Read the model definition and answer for the solid it produces. Units are mm, in the model's axes. A direction names the side the tool comes from. Give positions to 0.01 mm unless a question says otherwise; leave off trailing zeros. Order: outer loops, then holes, each group sorted by start corner. A loop starts at its lowest first (then second) coordinate and runs counter-clockwise, first axis right, second up. Notation, with made-up numbers: (36.5, -14) - (87.5, -14) arc R25 cw to (87.5, 2) - close; hole circle Ø5 at (-13, -7.75). An arc over 180 degrees is marked (long way). Write each question's results on one line, items separated by ' | '.
from build123d import *

# Parameters (mm, degrees)
BOSS_EXTRUDE1_DEPTH      = 1.5
BOSS_EXTRUDE1_DEPTH_BACK = 1.5
SKETCH1_R                = 8.5
SKETCH1_R_2              = 2.3
SKETCH2_W                = 3
SKETCH2_H                = 2.6
SKETCH2_W_2              = 2.6
SKETCH2_H_2              = 3
CUT_EXTRUDE1_DEPTH       = 13.389511693


with BuildPart() as part:
    # Sketch1 → Boss-Extrude1 (new, two sides: drawn at the far end of the back side and taken through both)
    with BuildSketch(Plane(origin=(0, 0, 0), x_dir=(1, 0, 0), z_dir=(0, 1, 0)).offset(-BOSS_EXTRUDE1_DEPTH_BACK)):
        with Locations(Location((0, 0, 0), (0, 0, 270))):
            Circle(SKETCH1_R)
        with Locations(Location((0, 0, 0), (0, 0, 270))):
            Circle(SKETCH1_R_2, mode=Mode.SUBTRACT)
    extrude(amount=BOSS_EXTRUDE1_DEPTH + BOSS_EXTRUDE1_DEPTH_BACK)

    # Sketch2 → Cut-Extrude1 (cut, through all)
    with BuildSketch(Plane(origin=(0, 1.5, 0), x_dir=(1, 0, 0), z_dir=(0, 1, 0))):
        with Locations((-7, 0)):
            Rectangle(SKETCH2_W, SKETCH2_H)
        with Locations((0, -7)):
            Rectangle(SKETCH2_W_2, SKETCH2_H_2)
        with Locations((0, 7)):
            Rectangle(SKETCH2_W_2, SKETCH2_H_2)
        with Locations((7, 0)):
            Rectangle(SKETCH2_W, SKETCH2_H)
    extrude(amount=-CUT_EXTRUDE1_DEPTH, mode=Mode.SUBTRACT)


solid = part.part
(1) Each of these flat-tipped pins is pushed along its axis until it touches: pin 1 (1.5 mm diameter, centred on x = -6.5, y = -0.5, fed in from +Z); pin 2 (0.8 mm diameter, centred on x = 0, y = -0.5, fed in from +Z); pin 3 (1.5 mm diameter, centred on y = 0, z = -6.5, fed in from +X). Where does it stop, or does it pass through?
Conclusion:
pin 1: z = 6.26 | pin 2: z = 5.5 | pin 3: x = 6.26
(2) The mould has two halves that part along X. Classify faces 6 (the face through (5.96, -0.02, 6.06)), 7 (the face through (-7, 0, -1.3)), 8 (the face through (1.3, 0, 7)), 9 (the face through (-5.96, -0.02, -6.06)): pulls with the +X half, pulls with the -X half, needs draft (parallel to the pull), parting line crosses it, or undercut.
Conclusion:
face 6: pulls with the +X half | face 7: needs draft | face 8: undercut | face 9: pulls with the -X half
(3) Section A-A (x = 0) is taken. Give the vertices of the cut face in (y, z), plus the area to 3 significant figures.
Conclusion:
outline: (-1.5, -5.5) - (1.5, -5.5) - (1.5, -2.3) - (-1.5, -2.3) - close; (-1.5, 2.3) - (1.5, 2.3) - (1.5, 5.5) - (-1.5, 5.5) - close | area: 19.2 mm^2
(4) Section B-B (z = 0) is taken. Give the vertices of the cut face in (x, y).
Conclusion:
outline: (-5.5, -1.5) - (-2.3, -1.5) - (-2.3, 1.5) - (-5.5, 1.5) - close; (2.3, -1.5) - (5.5, -1.5) - (5.5, 1.5) - (2.3, 1.5) - close
(5) Section C-C (y = -1.1) is taken. Give the vertices of the cut face in (x, z), plus the area to 3 significant figures.
Conclusion:
outline: (-8.4, -1.3) arc R8.5 ccw to (-1.3, -8.4) - (-1.3, -5.5) - (1.3, -5.5) - (1.3, -8.4) arc R8.5 ccw to (8.4, -1.3) - (5.5, -1.3) - (5.5, 1.3) - (8.4, 1.3) arc R8.5 ccw to (1.3, 8.4) - (1.3, 5.5) - (-1.3, 5.5) - (-1.3, 8.4) arc R8.5 ccw to (-8.4, 1.3) - (-5.5, 1.3) - (-5.5, -1.3) - close; hole circle Ø4.6 at (0, 0) | area: 180 mm^2
(6) For faces 1 (the face through (7, 0, 1.3)), 2 (the face through (0, 0, -5.5)), 3 (the face through (-5.5, 0, 0)), 4 (the face through (-1.3, 0, 7)), 5 (the face through (0.691, -0.021, 2.194)), determine the directions among +Z, -Z, +X, -X, +Y, -Y from which every point of the face is accessible in a straight line to the end or side of a thin tool.
Conclusion:
face 1: +X, +Y, -Y | face 2: -Z, +Y, -Y | face 3: -X, +Y, -Y | face 4: +Z, +Y, -Y | face 5: +Y, -Y
(7) Consider probe 1 along X at (y, z) = (-0.15, 0); probe 2 along Z at (x, y) = (-7, -1.05); probe 3 along X at (y, z) = (-0.4, -0.5) (3 decimals). Determine where each line is inside the solid, lowest interval first. Write a range as [from, to].
Conclusion:
probe 1: [-5.5, -2.3], [2.3, 5.5] | probe 2: [-4.82, -1.3], [1.3, 4.82] | probe 3: [-5.5, -2.245], [2.245, 5.5]
(8) Section D-D (x = 4.75) is taken. Give the vertices of the cut face in (y, z).
Conclusion:
outline: (-1.5, -7.05) - (1.5, -7.05) - (1.5, 7.05) - (-1.5, 7.05) - close
